Design review of the part built by this model. Coordinates are the model's own, in mm. A direction names the side the tool comes from. Give positions to 0.01 mm unless a question says otherwise; leave off trailing zeros. One line per item, written item: value.
from build123d import *

# Parameters (mm, degrees)
IZIM2_OUTSIDE_W                      = 120.946
IZIM2_OUTSIDE_H                      = 120.946
KES_EKSTR_ZYON1_DEPTH                = 40
IZIM3_OUTSIDE_W                      = 84.664
IZIM3_OUTSIDE_H                      = 54.164
KES_EKSTR_ZYON2_DEPTH                = 30
Y_KSEKLIK_EKSTR_ZYON2_START          = 9
IZIM11_R                             = 10.5
Y_KSEKLIK_EKSTR_ZYON2_DEPTH          = 9
M8X1_25_DI_LI_DELIK1_D               = 6.8
M8X1_25_DI_LI_DELIK1_DEPTH           = 18
M8X1_25_DI_LI_DELIK1_TIP             = 2.042926105
M8X1_25_DI_LI_DELIK2_D               = 6.8
M8X1_25_DI_LI_DELIK2_DEPTH           = 12
M8X1_25_DI_LI_DELIK2_TIP             = 2.042926105
M8X1_25_DI_LI_DELIK2_ON_FACE_2_D     = 6.8
M8X1_25_DI_LI_DELIK2_ON_FACE_2_DEPTH = 12
M8X1_25_DI_LI_DELIK2_ON_FACE_2_TIP   = 2.042926105
KES_EKSTR_ZYON3_DEPTH                = 7


with BuildPart() as part:
    # Çizim1 → Döndür1 (revolve)
    with BuildSketch(Plane.XY, mode=Mode.PRIVATE) as d_nd_r1_sk:
        with BuildLine():
            Line((0, -35), (0, -18))
            Line((0, -18), (8.5, -18))
            Line((8.5, -18), (8.5, -9))
            Line((8.5, -9), (10.5, -9))
            Line((10.5, -9), (10.5, -0.5))
            Line((10.5, -0.5), (11, 0))
            Line((11, 0), (11.5, 0))
            ThreePointArc((11.5, 0), (15.803393463, -2.321536849), (19.572591816, -5.436319733))
            ThreePointArc((19.572591816, -5.436319733), (29.328522406, -11.988638081), (40.852954694, -14.290489038))
            Line((40.852954694, -14.290489038), (46, -14.290489038))
            Line((46, -14.290489038), (46, -35))
            Line((46, -35), (0, -35))
        make_face()
    revolve(d_nd_r1_sk.sketch.rotate(Axis((0, 4.884743134, 0), (0, -1, 0)), 90), axis=Axis((0, 4.884743134, 0), (0, -1, 0)))

    # Çizim2 outside → Kes-Ekstrüzyon1 (cut)
    with BuildSketch(Plane(origin=(0, 0, 0), x_dir=(1, 0, 0), z_dir=(0, 1, 0))):
        Rectangle(IZIM2_OUTSIDE_W, IZIM2_OUTSIDE_H)
        with BuildLine():
            Line((-19.5, 11.5), (-19.5, -11.5))
            ThreePointArc((-19.5, -11.5), (-16.571067812, -18.571067812), (-9.5, -21.5))
            Line((-9.5, -21.5), (24.5, -21.5))
            ThreePointArc((24.5, -21.5), (46, 0), (24.5, 21.5))
            Line((24.5, 21.5), (-9.5, 21.5))
            ThreePointArc((-9.5, 21.5), (-16.571067812, 18.571067812), (-19.5, 11.5))
        make_face(mode=Mode.SUBTRACT)
    extrude(amount=-KES_EKSTR_ZYON1_DEPTH, mode=Mode.SUBTRACT)

    # Çizim3 outside → Kes-Ekstrüzyon2 (cut, symmetric)
    with BuildSketch(Plane.XY):
        with Locations((13.25, -17.5)):
            Rectangle(IZIM3_OUTSIDE_W, IZIM3_OUTSIDE_H)
        with BuildLine():
            Line((-19.5, -13), (-19.5, -5.36356579))
            ThreePointArc((-19.5, -5.36356579), (-15.760740466, -2.292876744), (-11.5, 0))
            Line((-11.5, 0), (11.5, 0))
            ThreePointArc((11.5, 0), (15.803393463, -2.321536849), (19.572591816, -5.436319733))
            ThreePointArc((19.572591816, -5.436319733), (29.328522406, -11.988638081), (40.852954694, -14.290489038))
            Line((40.852954694, -14.290489038), (46, -14.290489038))
            Line((46, -14.290489038), (46, -16.000690448))
            Line((46, -16.000690448), (-7.993980308, -32.508306842))
            ThreePointArc((-7.993980308, -32.508306842), (-9.31172617, -32.456532466), (-10.310774525, -31.59569733))
            Line((-10.310774525, -31.59569733), (-18.160254038, -18))
            ThreePointArc((-18.160254038, -18), (-19.159258263, -15.588190451), (-19.5, -13))
        make_face(mode=Mode.SUBTRACT)
    extrude(amount=KES_EKSTR_ZYON2_DEPTH, both=True, mode=Mode.SUBTRACT)

    # Çizim11 → Yükseklik-Ekstrüzyon2 (add)
    with BuildSketch(Plane(origin=(0, -18, 0), x_dir=(1, 0, 0), z_dir=(0, 1, 0)).offset(Y_KSEKLIK_EKSTR_ZYON2_START)):
        with Locations(Location((0, 0, 0), (0, 0, 270))):
            Circle(IZIM11_R)
    extrude(amount=-Y_KSEKLIK_EKSTR_ZYON2_DEPTH)

    # M8x1.25 Dişli Delik1
    with Locations(Plane(origin=(-0.844028469, -30.322347194, 0), x_dir=(-0.956304755963, -0.292371704723, 0), z_dir=(0.292371704723, -0.956304755963, 0))):
        with Locations((0, 0)):
            Hole(M8X1_25_DI_LI_DELIK1_D / 2, depth=M8X1_25_DI_LI_DELIK1_DEPTH)
            with Locations((0, 0, -(M8X1_25_DI_LI_DELIK1_DEPTH + M8X1_25_DI_LI_DELIK1_TIP / 2))):  # 118° drill point
                Cone(0, M8X1_25_DI_LI_DELIK1_D / 2, M8X1_25_DI_LI_DELIK1_TIP, mode=Mode.SUBTRACT)

    # M8x1.25 Dişli Delik2
    with Locations(Plane(origin=(21.70506177, -23.428398469, 12.310096913), x_dir=(-0.956304755963, -0.292371704723, 0), z_dir=(0.292371704723, -0.956304755963, 0))):
        with Locations((0, 0)):
            Hole(M8X1_25_DI_LI_DELIK2_D / 2, depth=M8X1_25_DI_LI_DELIK2_DEPTH)
            with Locations((0, 0, -(M8X1_25_DI_LI_DELIK2_DEPTH + M8X1_25_DI_LI_DELIK2_TIP / 2))):  # 118° drill point
                Cone(0, M8X1_25_DI_LI_DELIK2_D / 2, M8X1_25_DI_LI_DELIK2_TIP, mode=Mode.SUBTRACT)

    # M8x1.25 Dişli Delik2 on face 2
    with Locations(Plane(origin=(21.70506177, -23.428398469, -12.310096913), x_dir=(-0.956304694265, -0.292371906527, 0), z_dir=(0.292371906527, -0.956304694265, 0))):
        with Locations((0, 0)):
            Hole(M8X1_25_DI_LI_DELIK2_ON_FACE_2_D / 2, depth=M8X1_25_DI_LI_DELIK2_ON_FACE_2_DEPTH)
            with Locations((0, 0, -(M8X1_25_DI_LI_DELIK2_ON_FACE_2_DEPTH + M8X1_25_DI_LI_DELIK2_ON_FACE_2_TIP / 2))):  # 118° drill point
                Cone(0, M8X1_25_DI_LI_DELIK2_ON_FACE_2_D / 2, M8X1_25_DI_LI_DELIK2_ON_FACE_2_TIP, mode=Mode.SUBTRACT)

    # Çizim16 → Kes-Ekstrüzyon3 (cut)
    with BuildSketch(Plane(origin=(8.405872106, -27.494368788, 0), x_dir=(0.956304755963042, 0.2923717047227155, 0), z_dir=(0.29237170472271556, -0.9563047559630421, 0))):
        with BuildLine():
            Line((-16.172544779, -8.831760866), (-16.172544779, -15.810096913))
            ThreePointArc((-16.172544779, -15.810096913), (-15.293865123, -17.931417256), (-13.172544779, -18.810096913))
            Line((-13.172544779, -18.810096913), (5.075092134, -18.810096913))
            ThreePointArc((5.075092134, -18.810096913), (7.556602709, -17.495951373), (7.864069249, -14.704833755))
            ThreePointArc((7.864069249, -14.704833755), (9.081050216, -7.955601822), (15.670169023, -6.053842714))
            ThreePointArc((15.670169023, -6.053842714), (23.208480374, -0.112690383), (15.891078456, 6.098513866))
            ThreePointArc((15.891078456, 6.098513866), (15.779783551, 6.080333222), (15.670169023, 6.053842714))
            ThreePointArc((15.670169023, 6.053842714), (9.081050216, 7.955601822), (7.864069249, 14.704833755))
            ThreePointArc((7.864069249, 14.704833755), (7.556602709, 17.495951374), (5.075092134, 18.810096913))
            Line((5.075092134, 18.810096913), (-13.172544779, 18.810096913))
            ThreePointArc((-13.172544779, 18.810096913), (-15.293865123, 17.931417256), (-16.172544779, 15.810096913))
            Line((-16.172544779, 15.810096913), (-16.172544779, 8.831760866))
            ThreePointArc((-16.172544779, 8.831760866), (-14.85839924, 6.350250291), (-12.067281621, 6.042783751))
            ThreePointArc((-12.067281621, 6.042783751), (-3.172544779, 0), (-12.067281621, -6.042783751))
            ThreePointArc((-12.067281621, -6.042783751), (-14.85839924, -6.350250291), (-16.172544779, -8.831760866))
        make_face()
    extrude(amount=-KES_EKSTR_ZYON3_DEPTH, mode=Mode.SUBTRACT)


solid = part.part
Item 1: Machinability: for faces 4 (the flat face through (-8.07, -28.92, -12.27)), 5 (the conical face through (17.4, -10.43, 11.81)), 6 (the flat face through (0, -9, 0)), which of the approach directions +Z, -Z, +X, -X, +Y, -Y give a long, thin tool a straight path to every point of the face, cutting with its end or side? Answer none if there is none.
Returned:
face 4: +X
face 5: none
face 6: +Y
Item 2: Add section A-A on y = -17. Count the separate pieces of the cut face and the enclosed holes in it, plus the area to 3 significant figures.
Returned:
separate pieces: 1
enclosed holes: 4
area: 2,270 mm²
Item 3: Draft analysis for pull direction X (two halves, no side actions). For faces 1 (the cylindrical face through (29.587, -17.41, -0.266)), 2 (the flat face through (3, -20, 21.5)), 3 (the flat face through (-8.07, -28.92, 12.37)), state which applies: pulls with the +X half, pulls with the -X half, needs draft (parallel to the pull), parting line crosses it, or undercut.
Returned:
face 1: undercut
face 2: needs draft
face 3: pulls with the +X half
Item 4: To check wall thickness, follow line 1 along Z through (x, y) = (17, -15.5); line 2 along Z through (x, y) = (-1, -26.5); line 3 along X through (y, z) = (-5, -1.5). State the ranges of each line that lie inside material, in increasing order. Write a range as from..to.
Returned:
line 1: -21.5..-14.92, -9.7..9.7, 14.92..21.5
line 2: -21.5..-18.81, -6.43..-3.26, 3.26..6.43, 18.81..21.5
line 3: -19.07..-10.39, 10.39..19.07
Item 5: Clearance check with flat-ended pins moving along their axes: P1, Ø12, axis at y = -14, z = 15, coming from the +X side; P2, Ø3, axis at x = 24.5, z = 4.5, coming from the +Y side; P3, Ø1.5, axis at y = -17, z = 14, coming from the -X side. State where each tip first meets the part, or that it passes through.
Returned:
P1: x = 44.02
P2: y = -8.7
P3: x = -18.96
